```python
from build123d import *

# Parameters (mm, degrees)
SKETCH_1_R      = 1
EXTRUDE_1_DEPTH = 1.4


with BuildPart() as part:
    # 草图1 → 拉伸1 (new body)
    with BuildSketch(Plane(origin=(0, 0, 0), x_dir=(1, 0, 0), z_dir=(0, 1, 0))):
        with BuildLine():
            Line((-1.704686201, 10.867108399), (-2.036847592, 12.839441261))
            ThreePointArc((-2.036847592, 12.839441261), (4.873981347, -12.051734557), (-7.461076693, 10.64576604))
            Line((-7.461076693, 10.64576604), (-6.275343529, 9.034382303))
            ThreePointArc((-6.275343529, 9.034382303), (-6.193868184, 7.053393202), (-8.070099598, 6.412525252))
            ThreePointArc((-8.070099598, 6.412525252), (-8.711183181, 6.403482512), (-9.215009926, 6.006961967))
            ThreePointArc((-9.215009926, 6.006961967), (4.041226825, -10.230761739), (2.62241687, 10.682833414))
            ThreePointArc((2.62241687, 10.682833414), (1.978707932, 10.625847197), (1.504258862, 10.187091336))
            ThreePointArc((1.504258862, 10.187091336), (-0.354469436, 9.32728764), (-1.704686201, 10.867108399))
        make_face()
        with Locations(Location((0, 11, 0), (0, 0, 270))):
            Circle(SKETCH_1_R, mode=Mode.SUBTRACT)
        with Locations(Location((-7.561124809, 7.98932986, 0), (0, 0, 270))):
            Circle(SKETCH_1_R, mode=Mode.SUBTRACT)
    extrude(amount=EXTRUDE_1_DEPTH)


solid = part.part
```
Input: part model. Units: mm. Frame: model coordinates. A direction names the side the tool comes from. Give positions to 0.01 mm unless a question says otherwise; leave off trailing zeros. Order: outer loops, then holes, each group sorted by start corner. A loop starts at its lowest first (then second) coordinate and runs counter-clockwise, first axis right, second up.
1. Section C-C on y = 0.3. Return the cut outline in (x, z) (3 decimals), and give its area (3 significant figures).
Derived:
outline: (-9.215, -6.007) arc R11 cw (long way) to (2.622, -10.683) arc R1 cw to (1.504, -10.187) arc R1.71 ccw to (-1.705, -10.867) - (-2.037, -12.839) arc R13 ccw (long way) to (-7.461, -10.646) - (-6.275, -9.034) arc R1.657 ccw to (-8.07, -6.413) arc R1 cw to start; hole circle Ø2 at (-7.561, -7.989); hole circle Ø2 at (0, -11)
area: 143 mm2
2. Material intervals for L1, parallel to X at y = 0.9, z = 0; L2, parallel to Z at x = 0.5, y = 0.9; L3, parallel to X at y = 1.3, z = 5, sorted ascending.
Derived:
L1: x = -13 to -11, 11 to 13
L2: z = -12.99 to -11.87, -10.13 to -9.36, 10.99 to 12.99
L3: x = -12 to -9.8, 9.8 to 12
3. Mould query, pull axis X, two halves, no side actions, for faces 1 (the cylindrical face through (-0.32, 0.69, -9.32)), 2 (the cylindrical face through (-0.6, 0.7, -11.8)), 3 (the flat face through (-1.87, 0.69, -11.84)), 4 (the flat face through (1, 0, -10)). Classes: released by +X, released by -X, zero draft, split by the parting line, or undercut.
Derived:
face 1: undercut
face 2: undercut
face 3: released by -X
face 4: zero draft
4. Reachability of faces 5 (the flat face through (-6.877, 0.69, -9.851)), 6 (the cylindrical face through (1.99, 0.69, -10.63)), 7 (the flat face through (1, 1.4, -10)) from +Z, -Z, +X, -X, +Y, -Y: full face, straight path, thin tool, end or side. Return the list, or none.
Derived:
face 5: -Z, +Y, -Y
face 6: +Y, -Y
face 7: +Z, -Z, +X, -X, +Y
5. Section B-B on x = 0. Return the cut outline in (y, z).
Derived:
outline: (0, -13) - (1.4, -13) - (1.4, -12) - (0, -12) - close; (0, -10) - (1.4, -10) - (1.4, -9.29) - (0, -9.29) - close; (0, 11) - (1.4, 11) - (1.4, 13) - (0, 13) - close
6. Section D-D on x = 10.25. Return the cut outline in (y, z), and give its area (3 significant figures).
Derived:
outline: (0, -8) - (1.4, -8) - (1.4, -3.99) - (0, -3.99) - close; (0, 3.99) - (1.4, 3.99) - (1.4, 8) - (0, 8) - close
area: 11.2 mm2
7. Section A-A on z = 0. Return the cut outline in (x, y), and give its area (3 significant figures).
Derived:
outline: (-13, 0) - (-11, 0) - (-11, 1.4) - (-13, 1.4) - close; (11, 0) - (13, 0) - (13, 1.4) - (11, 1.4) - close
area: 5.60 mm2
